Read the model definition and answer for the solid it produces. Units are mm, in the model's axes. Give positions to 0.01 mm unless a question says otherwise; leave off trailing zeros. Order: outer loops, then holes, each group sorted by start corner. A loop starts at its lowest first (then second) coordinate and runs counter-clockwise, first axis right, second up. Notation, with made-up numbers: (46, 80) - (51, 80) arc R25 cw to (51, 96) - close; hole circle Ø5 at (-39.5, 62.25). An arc over 180 degrees is marked (long way). Return JSON: item names as keys, results as strings.
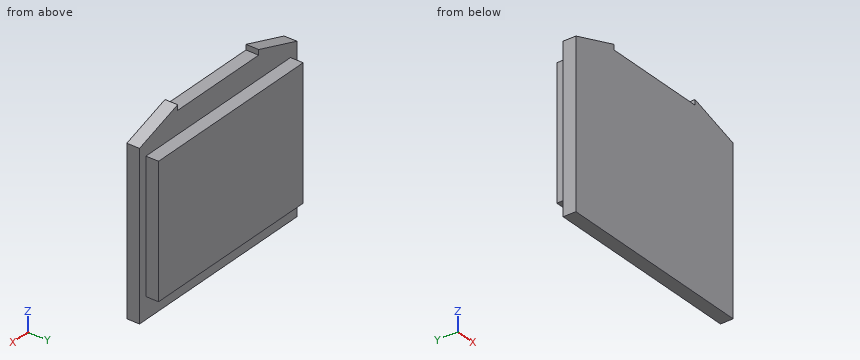
```python
from build123d import *

# Parameters (mm, degrees)
BOSS_EXTRUDE1_DEPTH = 1.7
SKETCH2_W           = 25
SKETCH2_H           = 17.5
BOSS_EXTRUDE2_DEPTH = 1.7
CHAMFER1_SIZE       = 12
CHAMFER1_SIZE_2     = 4
CHAMFER2_SIZE       = 4
CHAMFER2_SIZE_2     = 12
SKETCH3_W           = 27.2
SKETCH3_H           = 2.622019417
CUT_EXTRUDE1_DEPTH  = 20.771507277


with BuildPart() as part:
    # Sketch1 → Boss-Extrude1 (new body)
    with BuildSketch(Plane(origin=(0, 0, 0), x_dir=(1, 0, 0), z_dir=(0, 1, 0))):
        Polygon((-13.6, -14.25), (-7, -14.25), (-7, -11.75), (7, -11.75), (7, -14.25), (13.6, -14.25), (13.6, 14.25), (-13.6, 14.25), align=None)
    extrude(amount=BOSS_EXTRUDE1_DEPTH)

    # Sketch2 → Boss-Extrude2 (add)
    with BuildSketch(Plane(origin=(0, 1.7, 0), x_dir=(1, 0, 0), z_dir=(0, 1, 0))):
        Rectangle(SKETCH2_W, SKETCH2_H)
    extrude(amount=BOSS_EXTRUDE2_DEPTH)

    # Chamfer1
    # the kernel refuses this chamfer: 12, 4 mm, written as the material it takes off along each edge
    with BuildSketch(Plane(origin=(-13.6, -31.140732128, 14.25), x_dir=(0.9999257509361694, 0, 0.012185754582199854), z_dir=(0, 1, 0))) as chamfer1_piece_1:
        Polygon((CHAMFER1_SIZE * 0.999925750936, CHAMFER1_SIZE * 0.0121857545822), (-CHAMFER1_SIZE_2 * 0.0121857545822, CHAMFER1_SIZE_2 * 0.999925750936), (0, 0), align=None)
    extrude(amount=63.981464256, mode=Mode.SUBTRACT)

    # Chamfer2
    # the kernel refuses this chamfer: 12, 4 mm, written as the material it takes off along each edge
    with BuildSketch(Plane(origin=(13.6, -31.140732128, 14.25), x_dir=(0.10902612017980688, 0, -0.9940388851139268), z_dir=(0, 1, 0))) as chamfer2_piece_1:
        Polygon((CHAMFER2_SIZE * 0.994038885114, CHAMFER2_SIZE * 0.10902612018), (-CHAMFER2_SIZE_2 * 0.10902612018, CHAMFER2_SIZE_2 * 0.994038885114), (0, 0), align=None)
    extrude(amount=63.981464256, mode=Mode.SUBTRACT)

    # Sketch3 → Cut-Extrude1 (cut, through all)
    with BuildSketch(Plane(origin=(0, 1.7, 0), x_dir=(1, 0, 0), z_dir=(0, 1, 0))):
        with Locations((0, 12.938990292)):
            Rectangle(SKETCH3_W, SKETCH3_H)
    extrude(amount=-CUT_EXTRUDE1_DEPTH, mode=Mode.SUBTRACT)


solid = part.part
```
Q1. A cutting plane is placed at C-C (z = -9.25). Write down the section's boundary in (x, y).
Values:
{"outline": "(-13.6, 0) - (13.6, 0) - (13.6, 1.7) - (-13.6, 1.7) - close"}
Q2. Given pin 1 (0.8 mm diameter, centred on y = 2.5, z = -4, fed in from +X); pin 2 (0.8 mm diameter, centred on x = -3.5, y = 2, fed in from -Z); pin 3 (1.9 mm diameter, centred on x = -6, y = 3, fed in from +Z); pin 4 (2 mm diameter, centred on y = 3, z = -3, fed in from -X), each flat-ended and moving along its own axis, determine where each tip first touches the part or whether it passes through.
Values:
{"pin 1": "stops at x = 12.5", "pin 2": "stops at z = -11.63", "pin 3": "stops at z = 8.75", "pin 4": "stops at x = -12.5"}
Q3. Consider L1, parallel to Z at x = 5.5, y = 2.7; L2, parallel to Y at x = -3.5, z = 10.75; L3, parallel to X at y = 2.45, z = 2.5. Determine where each line is inside the solid, lowest interval first.
Values:
{"L1": "z = -8.75 to 8.75", "L2": "y = 0 to 1.7", "L3": "x = -12.5 to 12.5"}
Q4. A cutting plane is placed at B-B (x = 4.75). Write down the section's boundary in (y, z), and give its area (3 significant figures).
Values:
{"outline": "(0, -11.63) - (1.7, -11.63) - (1.7, -8.75) - (3.4, -8.75) - (3.4, 8.75) - (1.7, 8.75) - (1.7, 11.75) - (0, 11.75) - close", "area": "69.5 mm²"}
Q5. A cutting plane is placed at A-A (y = 0.4). Write down the section's boundary in (x, z), and give its area (3 significant figures).
Values:
{"outline": "(-13.6, -11.63) - (13.6, -11.63) - (13.6, 10.25) - (7, 12.45) - (7, 11.75) - (-7, 11.75) - (-7, 12.45) - (-13.6, 10.25) - close", "area": "631 mm²"}
Q6. A cutting plane is placed at D-D (y = 3.05). Write down the section's boundary in (x, z), and give its area (4 significant figures).
Values:
{"outline": "(-12.5, -8.75) - (12.5, -8.75) - (12.5, 8.75) - (-12.5, 8.75) - close", "area": "437.5 mm²"}
